For this review, use the dimensioned drawing (mm, ordinates from the lowest corner) and the shaded views. Give positions to 0.01 mm unless a question says otherwise; leave off trailing zeros. Write each loop counter-clockwise with the first axis right and the second up, starting at its lowest first coordinate (ties: lowest second). Pieces come first, ordered by that corner, then holes.
1) Wall thickness on line 1 along Y through (x, z) = (28, 1.25); line 2 along X through (y, z) = (22, 8); line 3 along Y through (x, z) = (18.5, 6.5): over which ranges is each line inside the solid? List them lowest first.
2) For P1, Ø0.9, axis at y = 32.5, z = 7, coming from the -X side; P2, Ø0.9, axis at x = 13, z = 7, coming from the -Y side; P3, Ø0.6, axis at y = 40, z = 4, coming from the +X side, all flat-tipped, find the tip position at first contact; note any pin that passes through.
3) We need section D-D on x = 11.5. Give the boundary of the cut face in (y, z), and give its area (3 significant figures).
4) We need section C-C on z = 6.25. Give the boundary of the cut face in (x, y), and give its area (3 significant figures).
5) We need section B-B on x = 24. Give the boundary of the cut face in (y, z), and give its area (3 significant figures).
6) We need section A-A on y = 36.5. Give the boundary of the cut face in (x, z), and give its area (3 significant figures).
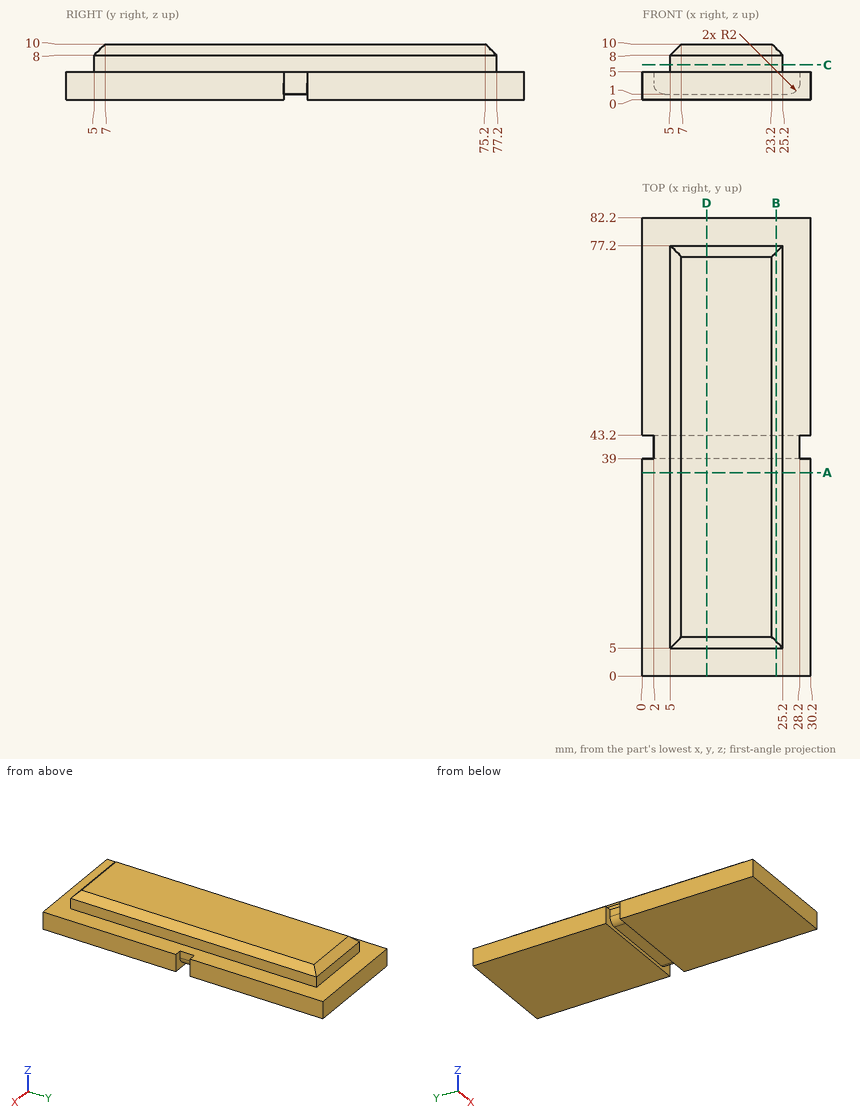
Results list:
1. line 1: y = 0 to 39, 43.2 to 82.2
1. line 2: x = 5 to 25.2
1. line 3: y = 5 to 77.2
2. P1: stops at x = 5
2. P2: stops at y = 5
2. P3: stops at x = 28.2
3. outline: (0, 0) - (39, 0) - (39, 1) - (43.2, 1) - (43.2, 0) - (82.2, 0) - (82.2, 5) - (77.2, 5) - (77.2, 8) - (75.2, 10) - (7, 10) - (5, 8) - (5, 5) - (0, 5) - close
3. area: 764 mm2
4. outline: (5, 5) - (25.2, 5) - (25.2, 77.2) - (5, 77.2) - close
4. area: 1,460 mm2
5. outline: (0, 0) - (39, 0) - (39, 1) - (43.2, 1) - (43.2, 0) - (82.2, 0) - (82.2, 5) - (77.2, 5) - (77.2, 8) - (76, 9.2) - (6.2, 9.2) - (5, 8) - (5, 5) - (0, 5) - close
5. area: 709 mm2
6. outline: (0, 0) - (30.2, 0) - (30.2, 5) - (25.2, 5) - (25.2, 8) - (23.2, 10) - (7, 10) - (5, 8) - (5, 5) - (0, 5) - close
6. area: 248 mm2
